CAD build for the part. Positions are in the model's coordinates, mm. Face numbers are marked on the shaded views. A direction names the side the tool comes from. Coordinates: 2 decimals unless noted, no trailing zeros. Order: outer loops, then holes, each group sorted by start corner. A loop starts at its lowest first (then second) coordinate and runs counter-clockwise, first axis right, second up. Notation, with made-up numbers: (-10, 23.5) - (6, 23.5) arc R13 ccw to (6, 31.5) - close; hole circle Ø9 at (-1, 75). An arc over 180 degrees is marked (long way). Return JSON: item names as keys, results as strings.
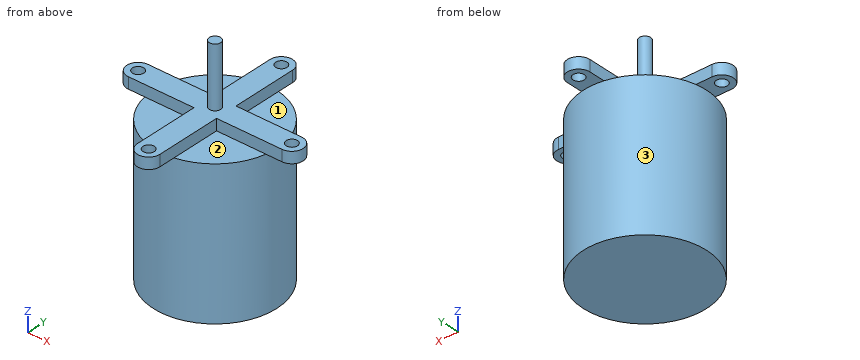
from build123d import *

# Parameters (mm, degrees)
SKETCH1_R           = 10.922
BOSS_EXTRUDE1_DEPTH = 25.654
SKETCH2_R           = 1.00000054
BOSS_EXTRUDE4_DEPTH = 2.00000108
SKETCH3_R           = 1.00000054
BOSS_EXTRUDE3_DEPTH = 12.7


with BuildPart() as part:
    # Sketch1 → Boss-Extrude1 (new body)
    with BuildSketch(Plane.XY):
        Circle(SKETCH1_R)
    extrude(amount=BOSS_EXTRUDE1_DEPTH)

    # Sketch2 → Boss-Extrude4 (add)
    # profile 1 of 7: a face of its own
    with BuildSketch(Plane.XY.offset(25.654)):
        with BuildLine():
            Line((-1.999996, 10.737322758), (-1.999996, 1.999996))
            Line((-1.999996, 1.999996), (1.999996, 1.999996))
            Line((1.999996, 1.999996), (1.999996, 10.737322758))
            ThreePointArc((1.999996, 10.737322758), (0, 10.922), (-1.999996, 10.737322758))
        make_face()
    # profile 2 of 7: a face of its own
    with BuildSketch(Plane.XY.offset(25.654)):
        with BuildLine():
            Line((-1.999996, 13.6118), (-1.999996, 10.737322758))
            ThreePointArc((-1.999996, 10.737322758), (0, 10.922), (1.999996, 10.737322758))
            Line((1.999996, 10.737322758), (1.999996, 13.6118))
            ThreePointArc((1.999996, 13.6118), (0, 15.611796), (-1.999996, 13.6118))
        make_face()
        with Locations((0, 13.6118)):
            Circle(SKETCH2_R, mode=Mode.SUBTRACT)
    # profile 3 of 7: a face of its own
    with BuildSketch(Plane.XY.offset(25.654)):
        with BuildLine():
            ThreePointArc((-10.737322758, 1.999996), (-10.922, 0), (-10.737322758, -1.999996))
            Line((-10.737322758, -1.999996), (-1.999996, -1.999996))
            Line((-1.999996, -1.999996), (-1.999996, -10.737322758))
            ThreePointArc((-1.999996, -10.737322758), (0, -10.922), (1.999996, -10.737322758))
            Line((1.999996, -10.737322758), (1.999996, -1.999996))
            Line((1.999996, -1.999996), (10.737322758, -1.999996))
            ThreePointArc((10.737322758, -1.999996), (10.875732692, -1.00425217), (10.922, 0))
            ThreePointArc((10.922, 0), (10.875732692, 1.00425217), (10.737322758, 1.999996))
            Line((10.737322758, 1.999996), (1.999996, 1.999996))
            Line((1.999996, 1.999996), (0, 0))
            Line((0, 0), (-1.999996, 1.999996))
            Line((-1.999996, 1.999996), (-10.737322758, 1.999996))
        make_face()
    # profile 4 of 7: a face of its own
    with BuildSketch(Plane.XY.offset(25.654)):
        with BuildLine():
            ThreePointArc((10.922, 0), (10.875732692, -1.00425217), (10.737322758, -1.999996))
            Line((10.737322758, -1.999996), (13.6118, -1.999996))
            ThreePointArc((13.6118, -1.999996), (15.611796, 0), (13.6118, 1.999996))
            Line((13.6118, 1.999996), (10.737322758, 1.999996))
            ThreePointArc((10.737322758, 1.999996), (10.875732692, 1.00425217), (10.922, 0))
        make_face()
        with Locations((13.6118, 0)):
            Circle(SKETCH2_R, mode=Mode.SUBTRACT)
    # profile 5 of 7: a face of its own
    with BuildSketch(Plane.XY.offset(25.654)):
        Polygon((1.999996, 1.999996), (-1.999996, 1.999996), (0, 0), align=None)
    # profile 6 of 7: a face of its own
    with BuildSketch(Plane.XY.offset(25.654)):
        with BuildLine():
            ThreePointArc((1.999996, -10.737322758), (0, -10.922), (-1.999996, -10.737322758))
            Line((-1.999996, -10.737322758), (-1.999996, -13.6118))
            ThreePointArc((-1.999996, -13.6118), (0, -15.611796), (1.999996, -13.6118))
            Line((1.999996, -13.6118), (1.999996, -10.737322758))
        make_face()
        with Locations((0, -13.6118)):
            Circle(SKETCH2_R, mode=Mode.SUBTRACT)
    # profile 7 of 7: a face of its own
    with BuildSketch(Plane.XY.offset(25.654)):
        with BuildLine():
            ThreePointArc((-13.6118, 1.999996), (-15.611796, 0), (-13.6118, -1.999996))
            Line((-13.6118, -1.999996), (-10.737322758, -1.999996))
            ThreePointArc((-10.737322758, -1.999996), (-10.922, 0), (-10.737322758, 1.999996))
            Line((-10.737322758, 1.999996), (-13.6118, 1.999996))
        make_face()
        with Locations((-13.6118, 0)):
            Circle(SKETCH2_R, mode=Mode.SUBTRACT)
    extrude(amount=BOSS_EXTRUDE4_DEPTH)

    # Sketch3 → Boss-Extrude3 (add)
    with BuildSketch(Plane.XY.offset(25.654)):
        Circle(SKETCH3_R)
    extrude(amount=BOSS_EXTRUDE3_DEPTH)


solid = part.part
Item 1: Drop flat-ended pins along their axis: P1, Ø1.6, axis at x = 8, z = 26.5, coming from the +Y side; P2, Ø1.6, axis at x = 7.5, z = 27, coming from the -Y side; P3, Ø12, axis at x = 8, z = 18, coming from the +Y side. Give the stop position or say it passes through.
Findings below:
{"P1": "stops at y = 2", "P2": "stops at y = -2", "P3": "stops at y = 10.74"}
Item 2: Band-saw the part on A-A, the plane y = 0. List the corners of the cut face in (x, z), then the cut area to 3 significant figures.
Findings below:
{"outline": "(-15.61, 25.65) - (-14.61, 25.65) - (-14.61, 27.65) - (-15.61, 27.65) - close; (-12.61, 25.65) - (-10.92, 25.65) - (-10.92, 0) - (10.92, 0) - (10.92, 25.65) - (12.61, 25.65) - (12.61, 27.65) - (1, 27.65) - (1, 38.35) - (-1, 38.35) - (-1, 27.65) - (-12.61, 27.65) - close; (14.61, 25.65) - (15.61, 25.65) - (15.61, 27.65) - (14.61, 27.65) - close", "area": "636 mm²"}
Item 3: Wall check: L1, parallel to Z at x = -0.5, y = 5; L2, parallel to Z at x = -5.5, y = -5.5; L3, parallel to X at y = -2, z = 25. Give the ranges that are in metal, low to high. Write a range as [from, to].
Findings below:
{"L1": "z = [0, 27.65]", "L2": "z = [0, 25.65]", "L3": "x = [-10.74, 10.74]"}
Item 4: Band-saw the part on C-C, the plane z = 33. List the corners of the cut face in (x, y).
Findings below:
{"outline": "circle Ø2 at (0, 0)"}
Item 5: Which spindle directions (+Z, -Z, +X, -X, +Y, -Y) get a long thin tool onto all of the face, cutting with end or side? Do the marked faces 1, 2 and 3. Say none if no direction does.
Findings below:
{"face 1": "+Z, +X, +Y", "face 2": "+Z, +X, -Y", "face 3": "-Z"}
Item 6: Band-saw the part on D-D, the plane y = 4. List the corners of the cut face in (x, z), then the cut area to 3 significant figures.
Findings below:
{"outline": "(-10.16, 0) - (10.16, 0) - (10.16, 25.65) - (2, 25.65) - (2, 27.65) - (-2, 27.65) - (-2, 25.65) - (-10.16, 25.65) - close", "area": "529 mm²"}
